Geometry check sheet. Reference: the model listing, model coordinates, mm. A direction names the side the tool comes from. Give positions to 0.01 mm unless a question says otherwise; leave off trailing zeros. Order: outer loops, then holes, each group sorted by start corner. A loop starts at its lowest first (then second) coordinate and runs counter-clockwise, first axis right, second up. Notation, with made-up numbers: M 52,52 L 107,52 A13 ccw 107,74 Z; hole C -29.75,-31 d3. An arc over 180 degrees is marked long. Answer as CSV lines item,"result". Start each with the question number.
```python
from build123d import *

# Parameters (mm, degrees)
F2_R     = 12.5
F3_DEPTH = 4.06
F4_R     = 1


with BuildPart() as f1:
    # F0 (on Front) → F1 (revolve)
    with BuildSketch(Plane.XZ):
        Polygon((-4.2, 8.575), (4.06, 8.575), (4.06, 11.18), (0, 11.18), (0, 11.63), (-4.2, 11.63), align=None)
    revolve(axis=Axis((0.086747, 0, 0), (-1, 0, 0)))

    # F2 (on Right) → F3 (cut, through all)
    with BuildSketch(Plane.YZ):
        Circle(F2_R)
        Polygon((-6.0438, 10.510589), (6.080537, 10.489379), (12.124337, -0.02121), (6.0438, -10.510589), (-6.080537, -10.489379), (-12.124337, 0.02121), align=None, mode=Mode.SUBTRACT)
    extrude(amount=F3_DEPTH, mode=Mode.SUBTRACT)

    # F4
    f4_edges = [f1.edges().sort_by_distance(p)[0] for p in [
        (-4.2, 0, -11.63),
    ]]
    fillet(f4_edges, radius=F4_R)


solid = f1.part
```
Item 1: Section check D-D on x = -0.75. Record the boundary of the cut face in (y, z) (3 decimals).
Item 2: Draft check along Z on faces 1 (the face through (2.002, 5.597, -9.678)), 2 (the face through (2.002, -5.597, 9.678)), 3 (the face through (4.06, -1, 9)), 4 (the face through (-0.012, 2.576, 8.179)). Enter one of: pulls with the +Z half, pulls with the -Z half, needs draft (parallel to the pull), parting line crosses it, or undercut.
Item 3: Access from +Z, -Z, +X, -X, +Y, -Y to the whole of each face (thin tool, end or side, straight path). Record for faces 5 (the face through (0, 9, 6)), 6 (the face through (2.002, 9.076, 5.281)), 7 (the face through (2, -9.11, 5.22)), 8 (the face through (2, 9.11, -5.22)), 9 (the face through (2, -5.58, -9.69)).
Item 4: Section check C-C on y = 0. Record the boundary of the cut face in (x, z) (3 decimals), then the cut area to 3 significant figures.
Item 5: Depth check by flat-ended pin: pin 1 Ø1 at (x, y) = (1, 7) entering from +Z; pin 2 Ø1.5 at (x, z) = (-1, -5.5) entering from +Y; pin 3 Ø4 at (x, y) = (1, 0.5) entering from +Z; pin 4 Ø1 at (x, y) = (2, 8) entering from -Z. Enter the tip coordinate at first touch or a pass-through.
Item 6: Section check A-A on z = 0. Record the boundary of the cut face in (x, y) (3 decimals).
Item 7: Scan lines: line 1 along Y through (x, z) = (0.5, 0) (3 decimals); line 2 along Y through (x, z) = (-0.75, 0) (3 decimals); line 3 along Z through (x, y) = (-3, -7.5). Record each from-to range of solid material in increasing order.
Item 8: Section check B-B on x = 1. Record the boundary of the cut face in (y, z) (3 decimals).
Numbers:
1,outline,"C 0,0 d23.26; hole C 0,0 d17.15"
2,face 1,"pulls with the -Z half"
2,face 2,"pulls with the +Z half"
2,face 3,"needs draft"
2,face 4,"undercut"
3,face 5,"+X"
3,face 6,"+Z, +X, +Y"
3,face 7,"+Z, +X, -Y"
3,face 8,"-Z, +X, +Y"
3,face 9,"-Z, +X, -Y"
4,outline,"M -4.2,-10.63 A1 ccw -3.2,-11.63 L 0,-11.63 L 0,-10.5 L 4.06,-10.5 L 4.06,-8.575 L -4.2,-8.575 Z; M -4.2,8.575 L 4.06,8.575 L 4.06,10.5 L 0,10.5 L 0,11.63 L -3.2,11.63 A1 ccw -4.2,10.63 Z"
4,area,"40.9 mm2"
5,pin 1,"z = 9.1"
5,pin 2,"y = 10.62"
5,pin 3,"z = 11.63"
5,pin 4,"z = -8"
6,outline,"M -4.2,-10.63 A1 ccw -3.2,-11.63 L 0,-11.63 L 0,-11.18 L 4.06,-11.18 L 4.06,-8.575 L -4.2,-8.575 Z; M -4.2,8.575 L 4.06,8.575 L 4.06,11.18 L 0,11.18 L 0,11.63 L -3.2,11.63 A1 ccw -4.2,10.63 Z"
7,line 1,"-11.18 to -8.575, 8.575 to 11.18"
7,line 2,"-11.63 to -8.575, 8.575 to 11.63"
7,line 3,"-8.89 to -4.16, 4.16 to 8.89"
8,outline,"M -11.016,-1.906 L -7.188,-8.563 A11.18 ccw -3.858,-10.493 L 3.821,-10.507 A11.18 ccw 7.158,-8.588 L 11.01,-1.944 A11.18 ccw 11.016,1.906 L 7.188,8.563 A11.18 ccw 3.858,10.493 L -3.821,10.507 A11.18 ccw -7.158,8.588 L -11.01,1.944 A11.18 ccw Z; hole C 0,0 d17.15"
